Read the model definition and answer for the solid it produces. Units are mm, in the model's axes. Give positions to 0.01 mm unless a question says otherwise; leave off trailing zeros. Order: outer loops, then holes, each group sorted by start corner. A loop starts at its lowest first (then second) coordinate and runs counter-clockwise, first axis right, second up.
Item 1: A cutting plane is placed at C-C (x = 30.5). Write down the section's boundary in (y, z), plus the area to 4 significant figures.
Item 2: Find the intervals of material crossed by line 1 along X through (y, z) = (4, 7.5); line 2 along Z through (x, y) = (6.25, 40); line 3 along Y through (x, z) = (3.5, 7.5), in increasing order.
Item 3: Given pin 1 Ø2.5 at (x, z) = (20, 7.5) entering from -Y; pin 2 Ø3 at (x, z) = (5, 7.5) entering from -Y; pin 3 Ø2.5 at (y, z) = (40, 7.5) entering from -X, each flat-ended and moving along its own axis, determine where each tip first touches the part or whether it passes through.
Item 4: A cutting plane is placed at D-D (y = 47.5). Write down the section's boundary in (x, z).
Item 5: A cutting plane is placed at A-A (z = 11). Write down the section's boundary in (x, y), plus the area to 3 significant figures.
Item 6: A cutting plane is placed at B-B (y = 7.5). Write down the section's boundary in (x, z).
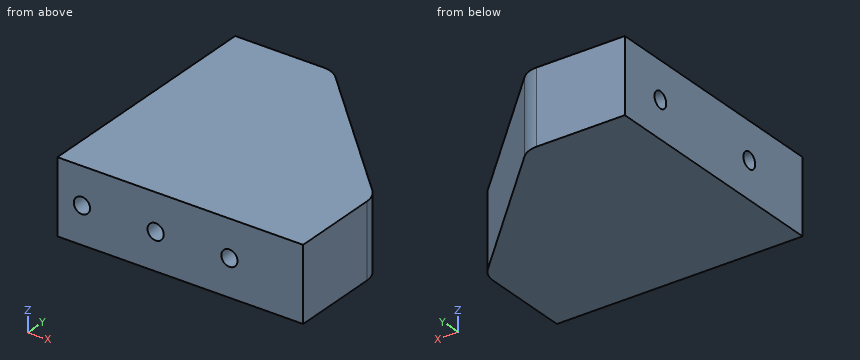
from build123d import *

# Parameters (mm, degrees)
BOSS_EXTRUDE1_DEPTH   = 15
M4_TAPPED_HOLE1_D     = 3.3
M4_TAPPED_HOLE1_DEPTH = 9.108579979
M4_TAPPED_HOLE1_TIP   = 0.991420021
M4_TAPPED_HOLE2_D     = 3.3
M4_TAPPED_HOLE2_DEPTH = 9.108579979
M4_TAPPED_HOLE2_TIP   = 0.991420021
FILLET1_R             = 5


with BuildPart() as part:
    # Sketch1 → Boss-Extrude1 (new body)
    with BuildSketch(Plane.XY):
        Polygon((0, 50), (20, 50), (50, 20), (50, 0), (0, 0), align=None)
    extrude(amount=BOSS_EXTRUDE1_DEPTH)

    # M4 Tapped Hole1
    with Locations(Plane(origin=(0, 40, 7.5), x_dir=(0, 0, -1), z_dir=(-1, 0, 0))):
        with Locations((0, 0), (0, 25)):
            Hole(M4_TAPPED_HOLE1_D / 2, depth=M4_TAPPED_HOLE1_DEPTH)
            with Locations((0, 0, -(M4_TAPPED_HOLE1_DEPTH + M4_TAPPED_HOLE1_TIP / 2))):  # 118° drill point
                Cone(0, M4_TAPPED_HOLE1_D / 2, M4_TAPPED_HOLE1_TIP, mode=Mode.SUBTRACT)

    # M4 Tapped Hole2
    with Locations(Plane(origin=(0, 0, 0), x_dir=(-1, 0, 0), z_dir=(0, -1, 0))):
        with Locations((-35, -7.5), (-20, -7.5), (-5, -7.5)):
            Hole(M4_TAPPED_HOLE2_D / 2, depth=M4_TAPPED_HOLE2_DEPTH)
            with Locations((0, 0, -(M4_TAPPED_HOLE2_DEPTH + M4_TAPPED_HOLE2_TIP / 2))):  # 118° drill point
                Cone(0, M4_TAPPED_HOLE2_D / 2, M4_TAPPED_HOLE2_TIP, mode=Mode.SUBTRACT)

    # Fillet1
    fillet1_edges = [part.edges().sort_by_distance(p)[0] for p in [
        (20, 50, 7.5),
        (50, 20, 7.5),
    ]]
    fillet(fillet1_edges, radius=FILLET1_R)


solid = part.part
Response values:
1. outline: (0, 0) - (39.5, 0) - (39.5, 15) - (0, 15) - close
1. area: 592.5 mm2
2. line 1: x = 0 to 3.35, 6.65 to 18.35, 21.65 to 33.35, 36.65 to 50
2. line 2: z = 0 to 5.85, 9.15 to 15
2. line 3: y = 9.2 to 13.35, 16.65 to 38.35, 41.65 to 50
3. pin 1: stops at y = 9.35
3. pin 2: stops at y = 9.2
3. pin 3: stops at x = 9.35
4. outline: (0, 0) - (22.5, 0) - (22.5, 15) - (0, 15) - close
5. outline: (0, 0) - (50, 0) - (50, 17.93) arc R5 ccw to (48.54, 21.46) - (21.46, 48.54) arc R5 ccw to (17.93, 50) - (0, 50) - close
5. area: 2,050 mm2
6. outline: (0, 0) - (50, 0) - (50, 15) - (0, 15) - close; hole circle Ø3.3 at (5, 7.5); hole circle Ø3.3 at (20, 7.5); hole circle Ø3.3 at (35, 7.5)
